Here's the drawing with two shaded views (mm, measured from the low corner). I have some questions. A direction names the side the tool comes from. Coordinates: 2 decimals unless noted, no trailing zeros. Loops run counter-clockwise (first coordinate to the right, second up) from the corner with the lowest first, then second, coordinate; pieces in that order, holes last. Notation, with made-up numbers: (-38.5, 32) - (-30.5, 32) arc R24 cw to (-30.5, 48) - close; hole circle Ø11 at (-4.75, 51.25). An arc over 180 degrees is marked (long way). Use a Markdown table: item, result.
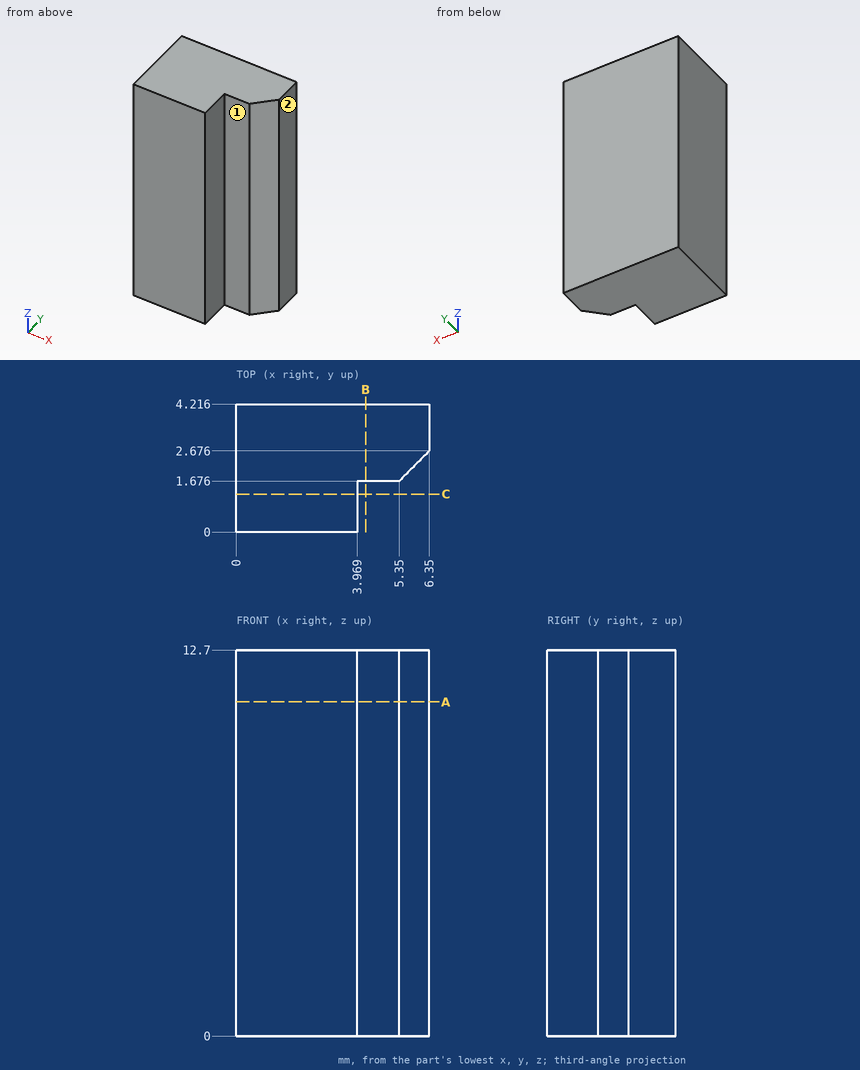
Q1. Which directions (+Z, -Z, +X, -X, +Y, -Y) give clear straight access to the entire face, cutting with the end or side of a thin tool? Please do the marked faces 1 and 2.
Check values:
| item | result |
|---|---|
| face 1 | +Z, -Z, +X, -Y |
| face 2 | +Z, -Z, +X, +Y, -Y |
Q2. I want a section at B-B, the plane x = 4.25. Write out the boundary of the cut face in (y, z).
Check values:
| item | result |
|---|---|
| outline | (1.68, 0) - (4.22, 0) - (4.22, 12.7) - (1.68, 12.7) - close |
Q3. Please list where these lines run through material, in increasing order: L1, parallel to X at y = 0.35, z = 1.25; L2, parallel to Y at x = 4.5, z = 1; L3, parallel to Y at x = 6, z = 4.5 (1 decimal). Write a range as from..to.
Check values:
| item | result |
|---|---|
| L1 | 0..3.97 |
| L2 | 1.68..4.22 |
| L3 | 2.3..4.2 |
Q4. I want a section at C-C, the plane y = 1.25. Write out the boundary of the cut face in (x, z).
Check values:
| item | result |
|---|---|
| outline | (0, 0) - (3.97, 0) - (3.97, 12.7) - (0, 12.7) - close |
Q5. I want a section at A-A, the plane z = 11. Write out the boundary of the cut face in (x, y), then the cut area to 3 significant figures.
Check values:
| item | result |
|---|---|
| outline | (0, 0) - (3.97, 0) - (3.97, 1.68) - (5.35, 1.68) - (6.35, 2.68) - (6.35, 4.22) - (0, 4.22) - close |
| area | 22.3 mm^2 |
